Can you work these out from the model? Positions are in its coordinate system, mm. Face numbers are marked on the shaded views. A direction names the side the tool comes from. Give positions to 0.01 mm unless a question says otherwise; leave off trailing zeros. Order: outer loops, then holes, each group sorted by start corner. A loop starts at its lowest first (then second) coordinate and runs counter-clockwise, first axis right, second up. Notation, with made-up numbers: M 18.5,61.25 L 35.5,61.25 A23 ccw 35.5,79.25 Z; hole C -23.5,-14.75 d2. An arc over 180 degrees is marked long. Answer as a JSON object with one key per item and string values.
```python
from build123d import *

# Parameters (mm, degrees)
SKETCH2_W           = 7.62
SKETCH2_H           = 8.89
SKETCH2_W_2         = 13.97
SKETCH2_H_2         = 44.45
BOSS_EXTRUDE1_DEPTH = 6.35
SKETCH3_R           = 4.0005
CUT_EXTRUDE1_DEPTH  = 2.794
CUT_EXTRUDE2_DEPTH  = 1.5875
CUT_EXTRUDE3_DEPTH  = 7.35


with BuildPart() as part:
    # Sketch2 → Boss-Extrude1 (new body)
    with BuildSketch(Plane.XY):
        with Locations((-17.78, 48.895)):
            Rectangle(SKETCH2_W, SKETCH2_H)
        with Locations((-6.985, 48.895)):
            Rectangle(SKETCH2_W_2, SKETCH2_H)
        with Locations((-6.985, 22.225)):
            Rectangle(SKETCH2_W_2, SKETCH2_H_2)
    extrude(amount=BOSS_EXTRUDE1_DEPTH)

    # Sketch3 → Cut-Extrude1 (cut)
    with BuildSketch(Plane(origin=(0, 0, 0), x_dir=(-1, 0, 0), z_dir=(0, 0, -1))):
        with Locations((6.985, 15.24)):
            Circle(SKETCH3_R)
    extrude(amount=-CUT_EXTRUDE1_DEPTH, mode=Mode.SUBTRACT)

    # Sketch4 → Cut-Extrude2 (cut)
    with BuildSketch(Plane(origin=(0, 0, 0), x_dir=(-1, 0, 0), z_dir=(0, 0, -1))):
        Polygon((6.985, 29.718), (9.017, 29.718), (9.017, 15.24), (9.017, 0.762), (4.953, 0.762), (4.953, 15.24), (4.953, 29.718), align=None)
    extrude(amount=-CUT_EXTRUDE2_DEPTH, mode=Mode.SUBTRACT)

    # Sketch5 → Cut-Extrude3 (cut, through all)
    with BuildSketch(Plane(origin=(0, 0, 0), x_dir=(-1, 0, 0), z_dir=(0, 0, -1))):
        Polygon((13.97, 44.45), (11.44430778, 44.45), (13.97, 26.791745209), align=None)
    extrude(amount=-CUT_EXTRUDE3_DEPTH, mode=Mode.SUBTRACT)


solid = part.part
```
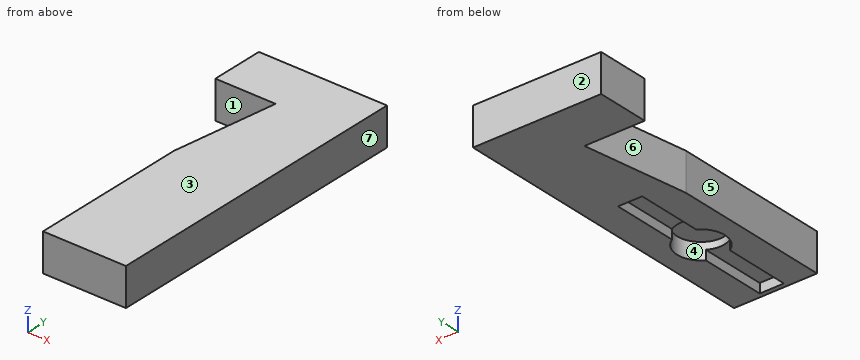
1) I need wall thicknesses on L1, parallel to Y at x = -16.75, z = 1; L2, parallel to X at y = 10.5, z = 5.5; L3, parallel to Z at x = -7.5, y = 29.5. Which ranges of each line are inside material? Lowest first, please.
Results found:
{"L1": "y = 44.45 to 53.34", "L2": "x = -13.97 to 0", "L3": "z = 1.59 to 6.35"}
2) I want a section at B-B on x = -6.75. Write out the boundary of the cut face in (y, z), and give its area (3 significant figures).
Results found:
{"outline": "M 0,0 L 0.76,0 L 0.76,1.59 L 11.25,1.59 L 11.25,2.79 L 19.23,2.79 L 19.23,1.59 L 29.72,1.59 L 29.72,0 L 53.34,0 L 53.34,6.35 L 0,6.35 Z", "area": "283 mm²"}
3) I want a section at C-C on y = 4.5. Write out the boundary of the cut face in (x, z).
Results found:
{"outline": "M -13.97,0 L -9.02,0 L -9.02,1.59 L -4.95,1.59 L -4.95,0 L 0,0 L 0,6.35 L -13.97,6.35 Z"}
4) I want a section at A-A on y = 15.24. Write out the boundary of the cut face in (x, z).
Results found:
{"outline": "M -13.97,0 L -10.99,0 L -10.99,2.79 L -2.98,2.79 L -2.98,0 L 0,0 L 0,6.35 L -13.97,6.35 Z"}
5) I want a section at D-D on x = -16.5. Write out the boundary of the cut face in (y, z).
Results found:
{"outline": "M 44.45,0 L 53.34,0 L 53.34,6.35 L 44.45,6.35 Z"}
6) Thinking about a two-plate mould opening in Y: for the marked faces 1, 2, 3 and 4, which applies, pulls with the +Y half, pulls with the -Y half, needs draft (parallel to the pull), parting line crosses it, or undercut?
Results found:
{"face 1": "undercut", "face 2": "pulls with the +Y half", "face 3": "needs draft", "face 4": "undercut"}
7) I'm going to push flat-ended pins straight in: pin 1 Ø1 at (y, z) = (18, 3.5) entering from -X; pin 2 Ø2.5 at (x, y) = (-6.5, 16) entering from -Z; pin 3 Ø3.5 at (x, y) = (-7, 7.5) entering from -Z. Where does each tip first touch, or does it pass through?
Results found:
{"pin 1": "stops at x = -13.97", "pin 2": "stops at z = 2.79", "pin 3": "stops at z = 1.59"}
8) For the marked faces 5, 6 and 7, which set-ups out of +Z, -Z, +X, -X, +Y, -Y let a thin tool reach every point of the face, with its end or its side?
Results found:
{"face 5": "+Z, -Z, -X, -Y", "face 6": "+Z, -Z, -X", "face 7": "+Z, -Z, +X, +Y, -Y"}
